CAD build for the part. Positions are in the model's coordinates, mm. Round coordinates to 2 decimals unless told otherwise and drop trailing zeros. Answer as a JSON object with one key per item and string values. Group by question number.
```python
from build123d import *

# Parameters (mm, degrees)
SKETCH1_W                  = 2.54
SKETCH1_H                  = 3.556
BOSS_EXTRUDE1_DEPTH        = 6.731
SKETCH2_W                  = 1.27
SKETCH2_H                  = 1.016
CUT_EXTRUDE1_DEPTH         = 5.461
CHAMFER1_SIZE              = 0.508
BOSS_EXTRUDE2_START        = -1.778
BOSS_EXTRUDE2_DEPTH        = 0.127
LPATTERN1_COUNT            = 12
LPATTERN1_PITCH            = 2.54
CHAMFER1_OF_LPATTERN1_SIZE = 0.508


with BuildPart() as part:
    # Sketch1 → Boss-Extrude1 (new body)
    with BuildSketch(Plane.XY):
        Rectangle(SKETCH1_W, SKETCH1_H)
    boss_extrude1 = extrude(amount=BOSS_EXTRUDE1_DEPTH)

    # Sketch2 → Cut-Extrude1 (cut)
    with BuildSketch(Plane.XY.offset(6.731)):
        Rectangle(SKETCH2_W, SKETCH2_H)
    cut_extrude1 = extrude(amount=-CUT_EXTRUDE1_DEPTH, mode=Mode.SUBTRACT)

    # Chamfer1
    chamfer1_edges = [part.edges().sort_by_distance(p)[0] for p in [
        (-0.635, 0, 6.731),
        (0, -0.508, 6.731),
        (0.635, 0, 6.731),
        (0, 0.508, 6.731),
    ]]
    chamfer(chamfer1_edges, length=CHAMFER1_SIZE)

    # Sketch3 → Boss-Extrude2 (add, symmetric)
    with BuildSketch(Plane(origin=(0, 1.778, 0), x_dir=(1, 0, 0), z_dir=(0, 1, 0)).offset(BOSS_EXTRUDE2_START)):
        Polygon((-0.381, 0), (-0.381, 2.667), (-0.1905, 3.175), (0.1905, 3.175), (0.381, 2.667), (0.381, 0), align=None)
    boss_extrude2 = extrude(amount=BOSS_EXTRUDE2_DEPTH, both=True)

    # LPattern1: Boss-Extrude1, Cut-Extrude1, Boss-Extrude2 ×12
    with Locations(*[(i * LPATTERN1_PITCH, 0, 0) for i in range(1, LPATTERN1_COUNT)]):
        add(boss_extrude1)
        add(cut_extrude1, mode=Mode.SUBTRACT)
        add(boss_extrude2)

    # Chamfer1 of LPattern1
    chamfer1_of_lpattern1_edges = [part.edges().sort_by_distance(p)[0] for p in [
        (1.905, 0, 6.731),
        (2.54, -0.508, 6.731),
        (3.175, 0, 6.731),
        (2.54, 0.508, 6.731),
        (4.445, 0, 6.731),
        (5.08, -0.508, 6.731),
        (5.715, 0, 6.731),
        (5.08, 0.508, 6.731),
        (6.985, 0, 6.731),
        (7.62, -0.508, 6.731),
        (8.255, 0, 6.731),
        (7.62, 0.508, 6.731),
        (9.525, 0, 6.731),
        (10.16, -0.508, 6.731),
        (10.795, 0, 6.731),
        (10.16, 0.508, 6.731),
        (12.065, 0, 6.731),
        (12.7, -0.508, 6.731),
        (13.335, 0, 6.731),
        (12.7, 0.508, 6.731),
        (14.605, 0, 6.731),
        (15.24, -0.508, 6.731),
        (15.875, 0, 6.731),
        (15.24, 0.508, 6.731),
        (17.145, 0, 6.731),
        (17.78, -0.508, 6.731),
        (18.415, 0, 6.731),
        (17.78, 0.508, 6.731),
        (19.685, 0, 6.731),
        (20.32, -0.508, 6.731),
        (20.955, 0, 6.731),
        (20.32, 0.508, 6.731),
        (22.225, 0, 6.731),
        (22.86, -0.508, 6.731),
        (23.495, 0, 6.731),
        (22.86, 0.508, 6.731),
        (24.765, 0, 6.731),
        (25.4, -0.508, 6.731),
        (26.035, 0, 6.731),
        (25.4, 0.508, 6.731),
        (27.305, 0, 6.731),
        (27.94, -0.508, 6.731),
        (28.575, 0, 6.731),
        (27.94, 0.508, 6.731),
    ]]
    chamfer(chamfer1_of_lpattern1_edges, length=CHAMFER1_OF_LPATTERN1_SIZE)


solid = part.part
```
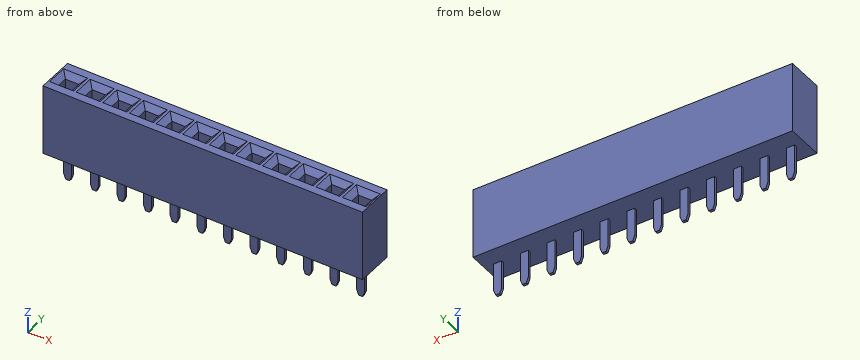
Item 1: Flat gauge pins, fed straight in: pin 1 Ø0.5 at (x, y) = (28, 0) entering from +Z; pin 2 Ø0.6 at (x, z) = (10.5, -1) entering from -Y. Where does each tip first touch, or does it go through?
Item 2: Drill centre lines: line 1 (Y direction, x = 17.5, z = 5.25); line 2 (Z direction, x = 24, y = 0.6); line 3 (Y direction, x = 12.5, z = -1). Where is each one in solid material? Low to high. Write a range as [from, to].
Item 3: Cut at A-A, the plane z = 2. Give the number of separate pieces and of enclosed holes in the cut face, and give its area (3 significant figures).
Response values:
{
 "1": {"pin 1": "z = 1.27", "pin 2": "y = -0.13"},
 "2": {"line 1": "[-1.78, -0.51], [0.51, 1.78]", "line 2": "[0, 6.73]", "line 3": "[-0.13, 0.13]"},
 "3": {"separate pieces": "1", "enclosed holes": "12", "area": "92.9 mm^2"}
}
